from build123d import *

# Parameters (mm, degrees)
SKETCH1_W           = 48.26
SKETCH1_H           = 6.35
SKETCH1_R           = 1.397
SKETCH1_R_2         = 1.4224
SKETCH1_R_3         = 1.4478
SKETCH1_R_4         = 1.4732
SKETCH1_R_5         = 1.4986
SKETCH1_R_6         = 1.524
SKETCH1_R_7         = 1.5494
SKETCH1_R_8         = 1.5748
SKETCH1_R_9         = 1.6002
BOSS_EXTRUDE1_DEPTH = 5.08
FILLET1_R           = 2.54


with BuildPart() as part:
    # Sketch1 → Boss-Extrude1 (new body)
    with BuildSketch(Plane(origin=(0, 0, 0), x_dir=(0, 1, 0), z_dir=(0, 0, 1))):
        with Locations((24.13, 3.175)):
            Rectangle(SKETCH1_W, SKETCH1_H)
        with Locations(Location((3.81, 3.175, 0), (0, 0, 270))):
            Circle(SKETCH1_R, mode=Mode.SUBTRACT)
        with Locations(Location((8.89, 3.175, 0), (0, 0, 270))):
            Circle(SKETCH1_R_2, mode=Mode.SUBTRACT)
        with Locations(Location((13.97, 3.175, 0), (0, 0, 270))):
            Circle(SKETCH1_R_3, mode=Mode.SUBTRACT)
        with Locations(Location((19.05, 3.175, 0), (0, 0, 270))):
            Circle(SKETCH1_R_4, mode=Mode.SUBTRACT)
        with Locations(Location((24.13, 3.175, 0), (0, 0, 270))):
            Circle(SKETCH1_R_5, mode=Mode.SUBTRACT)
        with Locations(Location((29.21, 3.175, 0), (0, 0, 270))):
            Circle(SKETCH1_R_6, mode=Mode.SUBTRACT)
        with Locations(Location((34.29, 3.175, 0), (0, 0, 270))):
            Circle(SKETCH1_R_7, mode=Mode.SUBTRACT)
        with Locations(Location((39.37, 3.175, 0), (0, 0, 270))):
            Circle(SKETCH1_R_8, mode=Mode.SUBTRACT)
        with Locations(Location((44.45, 3.175, 0), (0, 0, 270))):
            Circle(SKETCH1_R_9, mode=Mode.SUBTRACT)
    extrude(amount=BOSS_EXTRUDE1_DEPTH)

    # Fillet1
    fillet1_edges = [part.edges().sort_by_distance(p)[0] for p in [
        (-6.35, 0, 2.54),
    ]]
    fillet(fillet1_edges, radius=FILLET1_R)


solid = part.part
Input: part model. Units: mm. Frame: model coordinates. Give positions to 0.01 mm unless a question says otherwise; leave off trailing zeros. Write each loop counter-clockwise with the first axis right and the second up, starting at its lowest first coordinate (ties: lowest second). Pieces come first, ordered by that corner, then holes. Notation, with made-up numbers: (56, 3) -> (104, 3) arc R32 ccw to (104, 30) -> close; hole circle Ø8 at (84, -2.5). An arc over 180 degrees is marked (long way). Use one line per item in the form item = value. Start each with the question number.
1) Ray query, probe 1 along X at (y, z) = (28, 3.4); probe 2 along X at (y, z) = (15, 3.05); probe 3 along Y at (x, z) = (-5.25, 1.4). Return the intervals inside material, ascending. Write a range as from..to.
2) Section query B-B on z = 0.65. Count the separate pieces of the cut face and the enclosed holes in it, then the cut area to 3 significant figures.
3) Pin query (flat end, axial travel): pin 1 (3.5 mm diameter, centred on x = -3.175, y = 34.29, fed in from +Z); pin 2 (3 mm diameter, centred on x = -3.175, y = 44.45, fed in from +Z). Return the tip coordinate at first contact, or that it passes through.
4) Draft query along X for faces 1 (the flat face through (-5, 18, 0)), 2 (the cylindrical face through (-5.586, 0.724, 2.576)), 3 (the cylindrical face through (-4.317, 35.337, 2.504)). Return one class per face: pulls with the +X half, pulls with the -X half, needs draft (parallel to the pull), parting line crosses it, or undercut.
5) Section query C-C on y = 19.05. Return the cut outline in (x, z), then the cut area to 3 significant figures.
6) Section query A-A on y = 8.89. Return the cut outline in (x, z).
Outcome:
q1.probe_1 = -6.35..-4.1, -2.25..0
q1.probe_2 = -6.35..-4.19, -2.16..0
q1.probe_3 = 0.45..48.26
q2.separate_pieces = 1
q2.enclosed_holes = 9
q2.area = 241 mm^2
q3.pin_1 = 5.08
q3.pin_2 = through
q4.face_1 = needs draft
q4.face_2 = pulls with the -X half
q4.face_3 = undercut
q5.outline = (-6.35, 0) -> (-4.65, 0) -> (-4.65, 5.08) -> (-6.35, 5.08) -> close; (-1.7, 0) -> (0, 0) -> (0, 5.08) -> (-1.7, 5.08) -> close
q5.area = 17.3 mm^2
q6.outline = (-6.35, 0) -> (-4.6, 0) -> (-4.6, 5.08) -> (-6.35, 5.08) -> close; (-1.75, 0) -> (0, 0) -> (0, 5.08) -> (-1.75, 5.08) -> close
